from build123d import *

# Parameters (mm, degrees)
SKETCH1_W                                = 65
SKETCH1_H                                = 80
BOSS_EXTRUDE1_DEPTH                      = 5
SKETCH2_W                                = 65
SKETCH2_H                                = 80
SKETCH2_W_2                              = 57
SKETCH2_H_2                              = 72
BOSS_EXTRUDE2_DEPTH                      = 30
SKETCH3_R                                = 3.85
BOSS_EXTRUDE3_DEPTH                      = 20
TAP_DRILL_FOR_M3_TAP1_D                  = 2.5
TAP_DRILL_FOR_M3_TAP1_DEPTH              = 12
TAP_DRILL_FOR_M3_TAP1_TIP                = 0.751075774
CUT_EXTRUDE1_DEPTH                       = 2.7
MIRROR1_AT_THE_SECOND_PLANE_COPY_1_DEPTH = 2.7


with BuildPart() as part:
    # Sketch1 → Boss-Extrude1 (new body)
    with BuildSketch(Plane(origin=(0, 0, 0), x_dir=(1, 0, 0), z_dir=(0, 1, 0))):
        Rectangle(SKETCH1_W, SKETCH1_H)
    extrude(amount=BOSS_EXTRUDE1_DEPTH)

    # Sketch2 → Boss-Extrude2 (add)
    with BuildSketch(Plane(origin=(0, 5, 0), x_dir=(1, 0, 0), z_dir=(0, 1, 0))):
        Rectangle(SKETCH2_W, SKETCH2_H)
        Rectangle(SKETCH2_W_2, SKETCH2_H_2, mode=Mode.SUBTRACT)
    extrude(amount=BOSS_EXTRUDE2_DEPTH)

    # Sketch3 → Boss-Extrude3 (add)
    with BuildSketch(Plane(origin=(0, 5, 0), x_dir=(1, 0, 0), z_dir=(0, 1, 0))):
        with Locations(Location((-20.5, -28, 0), (0, 0, 90))):
            Circle(SKETCH3_R)
        with Locations(Location((20.5, -28, 0), (0, 0, 90))):
            Circle(SKETCH3_R)
        with Locations(Location((20.5, 28, 0), (0, 0, 90))):
            Circle(SKETCH3_R)
        with Locations(Location((-20.5, 28, 0), (0, 0, 90))):
            Circle(SKETCH3_R)
    extrude(amount=BOSS_EXTRUDE3_DEPTH)

    # Tap Drill for M3 Tap1
    with Locations(Plane(origin=(0, 25, 0), x_dir=(1, 0, 0), z_dir=(0, 1, 0))):
        with Locations((-20.5, 28), (20.5, 28), (20.5, -28), (-20.5, -28)):
            Hole(TAP_DRILL_FOR_M3_TAP1_D / 2, depth=TAP_DRILL_FOR_M3_TAP1_DEPTH)
            with Locations((0, 0, -(TAP_DRILL_FOR_M3_TAP1_DEPTH + TAP_DRILL_FOR_M3_TAP1_TIP / 2))):  # 118° drill point
                Cone(0, TAP_DRILL_FOR_M3_TAP1_D / 2, TAP_DRILL_FOR_M3_TAP1_TIP, mode=Mode.SUBTRACT)

    # Sketch8 → Cut-Extrude1 (cut)
    with BuildSketch(Plane(origin=(0, 25, 0), x_dir=(1, 0, 0), z_dir=(0, 1, 0))):
        Polygon((-17.382308546, 28), (-18.941154273, 30.7), (-22.058845727, 30.7), (-23.617691454, 28), (-22.058845727, 25.3), (-18.941154273, 25.3), align=None)
    cut_extrude1 = extrude(amount=-CUT_EXTRUDE1_DEPTH, mode=Mode.SUBTRACT)

    # Mirror1: Cut-Extrude1 across plane
    add(cut_extrude1.mirror(Plane.XY), mode=Mode.SUBTRACT)

    # Mirror1 at the second plane: Cut-Extrude1 across plane
    add(cut_extrude1.mirror(Plane(origin=(0, 0, 0), x_dir=(0, 0, 1), z_dir=(1, 0, 0))), mode=Mode.SUBTRACT)

    # Mirror1 at the second plane copy 1 sketc → Mirror1 at the second plane copy 1 (cut)
    with BuildSketch(Plane(origin=(0, 25, 0), x_dir=(-1, 0, 0), z_dir=(0, 1, 0))):
        Polygon((-17.382308546, 28), (-18.941154273, 30.7), (-22.058845727, 30.7), (-23.617691454, 28), (-22.058845727, 25.3), (-18.941154273, 25.3), align=None)
    extrude(amount=-MIRROR1_AT_THE_SECOND_PLANE_COPY_1_DEPTH, mode=Mode.SUBTRACT)


solid = part.part
Could you check a few things on this model? Use its own coordinates, in mm. Give positions to 0.01 mm unless a question says otherwise; leave off trailing zeros. Order: outer loops, then holes, each group sorted by start corner. A loop starts at its lowest first (then second) coordinate and runs counter-clockwise, first axis right, second up.
1. Suppose I cut it at B-B (y = 26.5). List the corners of the cut face in (x, z) for me, plus the area to 3 significant figures.
2. Will these pins go through, and if not, where does the flat tip stop? P1, Ø1.6, axis at x = -20, z = -27.5, coming from the +Y side; P2, Ø1.5, axis at x = -12.5, z = 19.5, coming from the +Y side; P3, Ø4.5, axis at x = 20, z = 29, coming from the +Y side.
3. Suppose I cut it at C-C (x = 27). List the corners of the cut face in (y, z) for me, plus the area to 3 significant figures.
4. Suppose I cut it at A-A (y = 17). Give the number of separate pieces and of enclosed holes in the cut face, plus the area to 3 significant figures.
5. Suppose I cut it at D-D (z = -17.5). List the corners of the cut face in (x, y) for me.
6. I need wall thicknesses on L1, parallel to Z at x = -20.5, y = 15; L2, parallel to X at y = 16, z = 28; L3, parallel to X at y = 18, z = -15. Which ranges of each line are inside material? Lowest first, please.
Solved:
1. outline: (-32.5, -40) - (32.5, -40) - (32.5, 40) - (-32.5, 40) - close; hole (-28.5, -36) - (28.5, -36) - (28.5, 36) - (-28.5, 36) - close
1. area: 1,100 mm2
2. P1: stops at y = 22.3
2. P2: stops at y = 5
2. P3: stops at y = 25
3. outline: (0, -40) - (35, -40) - (35, -36) - (5, -36) - (5, 36) - (35, 36) - (35, 40) - (0, 40) - close
3. area: 640 mm2
4. separate pieces: 5
4. enclosed holes: 5
4. area: 1,260 mm2
5. outline: (-32.5, 0) - (32.5, 0) - (32.5, 35) - (28.5, 35) - (28.5, 5) - (-28.5, 5) - (-28.5, 35) - (-32.5, 35) - close
6. L1: z = -40 to -36, -31.85 to -29.25, -26.75 to -24.15, 24.15 to 26.75, 29.25 to 31.85, 36 to 40
6. L2: x = -32.5 to -28.5, -24.35 to -21.75, -19.25 to -16.65, 16.65 to 19.25, 21.75 to 24.35, 28.5 to 32.5
6. L3: x = -32.5 to -28.5, 28.5 to 32.5
